Autodesk Inventor part; units mm, degrees
ref_plane "YZ Plane" through (0, 0, 0) normal (1, 0, 0) x (0, 1, 0)
ref_plane "XZ Plane" through (0, 0, 0) normal (0, 1, 0) x (-1, 0, 0)
ref_plane "XY Plane" through (0, 0, 0) normal (0, 0, 1) x (1, 0, 0)
sketch "Sketch1" plane through (0, 0, 0) normal (0, 0, 1) x (1, 0, 0)
  line L0 (-42.8625, -38.1) -> (-42.8625, 26.1937)
  arc A0 (6.35, 26.1938) -> (-42.8625, 26.1937) centre (-18.2562, 26.1937) ccw
  line L1 (6.35, 26.1938) -> (6.35, 15.875)
  line L2 (-39.6875, -38.1) -> (-39.6875, 26.1937)
  arc A1 (3.175, 26.1938) -> (-39.6875, 26.1937) centre (-18.2562, 26.1937) ccw
  line L3 (3.175, 26.1938) -> (3.175, 15.875)
  line L4 (-42.8625, -38.1) -> (-39.6875, -38.1)
  line L5 (3.175, 15.875) -> (6.35, 15.875)
  dimension "d0" = 3.175
  dimension "d1" = 88.9
  dimension "d2" = 21.4312
  dimension "d3" = 34.925
extrude "Extrusion1" add sketch "Sketch1" along normal blind 25.4
hole "Hole1" at (-39.6875, -31.75, 12.7) direction (-1, 0, 0) diameter 6.35 end through all
pattern_linear "Rectangular Pattern1" count 2 spacing 25.4 along (0, 1, 0) of "Hole1"
properties part number "FE-00016"
Verification items for the finished model (mm, model axes). A direction names the side the tool comes from. Coordinates: 2 decimals unless noted, no trailing zeros. Write each loop counter-clockwise with the first axis right and the second up, starting at its lowest first coordinate (ties: lowest second). Pieces come first, ordered by that corner, then holes. Notation, with made-up numbers: M 3.25,48 L 24.25,48 A27 ccw 24.25,85 Z; hole C -6.75,-35 d9. An arc over 180 degrees is marked long. Answer as a JSON object with one key per item and string values. Group by question number.
(1) Gauge pin test, flat ends, axial feed: pin 1 (6 mm diameter, centred on x = -11, z = 7, fed in from -Y); pin 2 (7.5 mm diameter, centred on y = 3.5, z = 18.5, fed in from +X); pin 3 (6 mm diameter, centred on x = -11.5, z = 9.5, fed in from -Y); pin 4 (5.5 mm diameter, centred on y = -6.35, z = 12.7, fed in from -X). Record the tip position at first contact, or that the pin passes through.
(2) Cross-section at A-A, the plane z = 12.7. State how many separate pieces and enclosed holes the cut face has, and give its area (3 significant figures).
(3) Material ranges on line 1 (Y direction, x = -40.9, z = 12.7) (3 decimals); line 2 (Y direction, x = -41, z = 12.7) (3 decimals); line 3 (X direction, y = 15, z = 12.75), recorded low to high.
(4) Cross-section at B-B, the plane y = -31.75. Record the cut outline in (x, z) (1 decimal).
(5) Tool access check on faces 5 (the face through (5, 15.875, 13)), 6 (the face through (-42.862, -6, 18)). Record the directions out of +Z, -Z, +X, -X, +Y, -Y that give a thin tool (end or side, any length) a straight path to the whole face; none if there is none.
(6) Cross-section at D-D, the plane y = -5. Record the cut outline in (x, z), and give its area (3 significant figures).
(7) Release check for a two-part mould opening along Z. For faces 1 (the face through (-41.3, -28.65, 13.39)), 2 (the face through (-40, 16, 25.4)), 3 (the face through (-41.297, -9.027, 10.993)), 4 (the face through (3.175, 21, 13)) record: +Z half, -Z half, draft (parallel to the pull), parting line (faces both ways), or undercut.
Reply:
{
 "1": {"pin 1": "y = 45.01", "pin 2": "x = -39.69", "pin 3": "y = 45.28", "pin 4": "through"},
 "2": {"separate pieces": "3", "enclosed holes": "0", "area": "426 mm²"},
 "3": {"line 1": "-38.1 to -34.925, -28.575 to -9.525, -3.175 to 35.823", "line 2": "-38.1 to -34.925, -28.575 to -9.525, -3.175 to 35.585", "line 3": "-42.86 to -39.69"},
 "4": {"outline": "M -42.9,0 L -39.7,0 L -39.7,9.5 L -42.9,9.5 Z; M -42.9,15.9 L -39.7,15.9 L -39.7,25.4 L -42.9,25.4 Z"},
 "5": {"face 5": "+Z, -Z, +X, -Y", "face 6": "+Z, -Z, -X, +Y, -Y"},
 "6": {"outline": "M -42.86,0 L -39.69,0 L -39.69,9.83 L -42.86,9.83 Z; M -42.86,15.57 L -39.69,15.57 L -39.69,25.4 L -42.86,25.4 Z", "area": "62.4 mm²"},
 "7": {"face 1": "undercut", "face 2": "+Z half", "face 3": "undercut", "face 4": "draft"}
}
